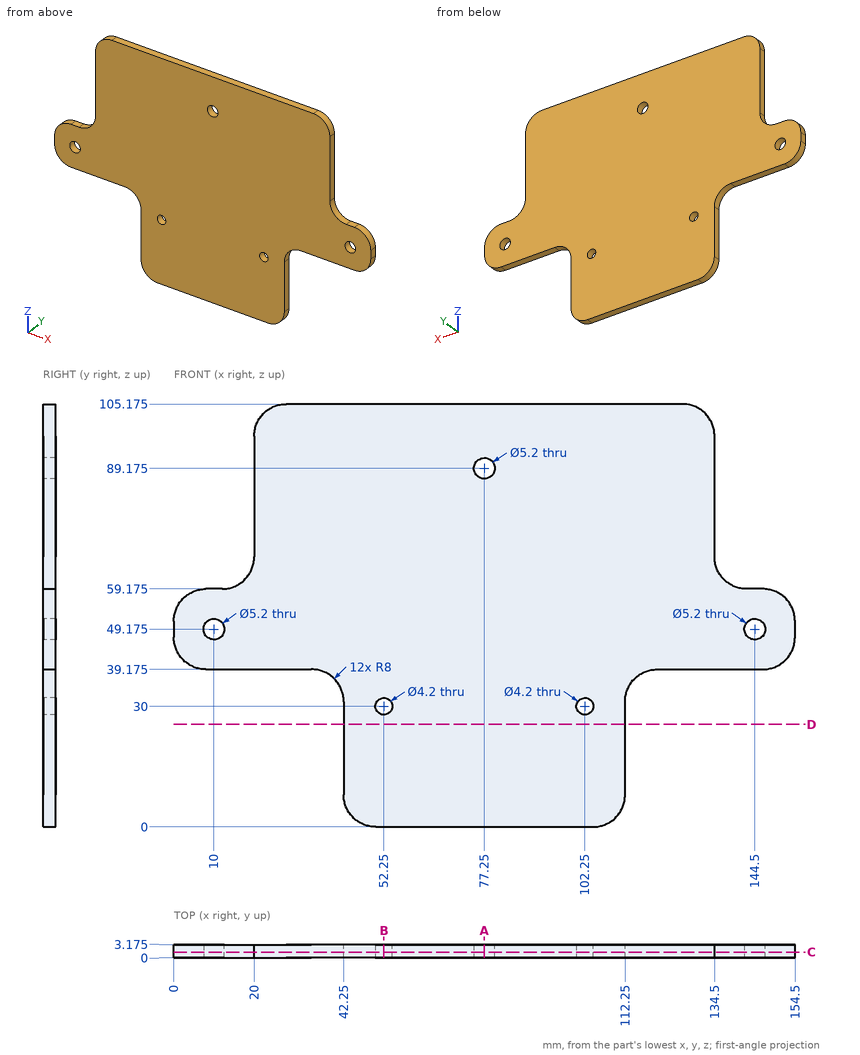
For this review, use the dimensioned drawing (mm, ordinates from the lowest corner) and the shaded views. Round coordinates to 2 decimals unless told otherwise and drop trailing zeros. Loops run counter-clockwise (first coordinate to the right, second up) from the corner with the lowest first, then second, coordinate; pieces in that order, holes last. Notation, with made-up numbers: M 46,20 L 99,20 A22 cw 99,34 Z; hole C 37,-30 d6. An arc over 180 degrees is marked long. Answer as a JSON object with one key per item and string values.
(1) Take a section at D-D on z = 25.5. Give the boundary of the cut face in (x, y) (3 decimals), and give its area (3 significant figures).
Resolved:
{"outline": "M 42.25,0 L 112.25,0 L 112.25,3.175 L 42.25,3.175 Z", "area": "222 mm²"}
(2) To check wall thickness, follow line 1 along X through (y, z) = (0.7, 30); line 2 along Z through (x, y) = (77.25, 0.8) (3 decimals); line 3 along Z through (x, y) = (52.25, 2.45) (3 decimals). State the ranges of each line that lie inside material, in increasing order.
Resolved:
{"line 1": "42.25 to 50.15, 54.35 to 100.15, 104.35 to 112.25", "line 2": "0 to 86.575, 91.775 to 105.175", "line 3": "0 to 27.9, 32.1 to 105.175"}
(3) Take a section at A-A on x = 77.25. Give the boundary of the cut face in (y, z) (3 decimals).
Resolved:
{"outline": "M 0,0 L 3.175,0 L 3.175,86.575 L 0,86.575 Z; M 0,91.775 L 3.175,91.775 L 3.175,105.175 L 0,105.175 Z"}
(4) Take a section at C-C on y = 1.35. Count the separate pieces of the cut face and the enclosed holes in it, and give its area (3 significant figures).
Resolved:
{"separate pieces": "1", "enclosed holes": "5", "area": "11,000 mm²"}
(5) Clearance check with flat-ended pins moving along their axes: P1, Ø1, axis at x = 134.5, y = 1, coming from the -Z side (3 decimals); P2, Ø1, axis at y = 2.5, z = 21.5, coming from the +X side. State where each tip first meets the part, or that it passes through.
Resolved:
{"P1": "z = 39.175", "P2": "x = 112.25"}
(6) Take a section at B-B on x = 52.25. Give the boundary of the cut face in (y, z) (3 decimals).
Resolved:
{"outline": "M 0,0 L 3.175,0 L 3.175,27.9 L 0,27.9 Z; M 0,32.1 L 3.175,32.1 L 3.175,105.175 L 0,105.175 Z"}
